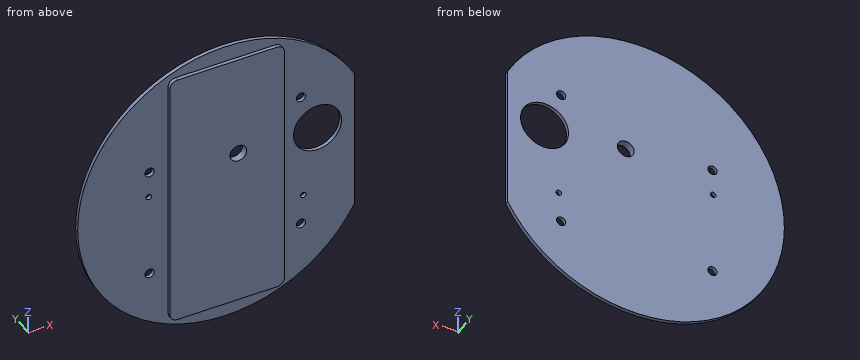
from build123d import *

# Parameters (mm, degrees)
F1_DEPTH  = 2
F2_W      = 62
F2_H      = 142.5
F3_DEPTH  = 2
F4_R      = 4
F5_R      = 4.5
F6_DEPTH  = 4
F7_R      = 13
F8_DEPTH  = 2
F9_R      = 2.5
F10_DEPTH = 2
F11_R     = 1.5
F12_DEPTH = 2


with BuildPart() as f1:
    # F0 (on Front) → F1 (new body)
    with BuildSketch(Plane.XZ):
        with BuildLine():
            ThreePointArc((70, 38.729833), (-80, 0), (70, -38.729833))
            Line((70, -38.729833), (70, 38.729833))
        make_face()
    extrude(amount=F1_DEPTH)

    # F2 (on face) → F3 (join)
    with BuildSketch(Plane.XZ.offset(2)):
        Rectangle(F2_W, F2_H)
    extrude(amount=F3_DEPTH)

    # F4
    f4_edges = [f1.edges().sort_by_distance(p)[0] for p in [
        (-31, -3, -71.25),
        (31, -3, -71.25),
        (31, -3, 71.25),
        (-31, -3, 71.25),
    ]]
    fillet(f4_edges, radius=F4_R)

    # F5 (on face) → F6 (cut)
    with BuildSketch(Plane.XZ.offset(4)):
        with Locations((6, 15.75)):
            Circle(F5_R)
    extrude(amount=-F6_DEPTH, mode=Mode.SUBTRACT)

    # F7 (on face) → F8 (cut)
    with BuildSketch(Plane.XZ.offset(2)):
        with Locations((50, 13.729833)):
            Circle(F7_R)
    extrude(amount=-F8_DEPTH, mode=Mode.SUBTRACT)

    # F9 (on face) → F10 (cut)
    with BuildSketch(Plane.XZ.offset(2)):
        with Locations((-41, 20)):
            Circle(F9_R)
        with Locations((-41, -40)):
            Circle(F9_R)
        with Locations((41, 35)):
            Circle(F9_R)
        with Locations((41, -40)):
            Circle(F9_R)
    extrude(amount=-F10_DEPTH, mode=Mode.SUBTRACT)

    # F11 (on face) → F12 (cut)
    with BuildSketch(Plane.XZ.offset(2)):
        with Locations((-41.405737, 5.505678)):
            Circle(F11_R)
        with Locations((42.2996, -23.55126)):
            Circle(F11_R)
    extrude(amount=-F12_DEPTH, mode=Mode.SUBTRACT)


solid = f1.part
Can you work these out from the model? Positions are in its coordinate system, mm. Coordinates: 2 decimals unless noted, no trailing zeros. Order: outer loops, then holes, each group sorted by start corner. A loop starts at its lowest first (then second) coordinate and runs counter-clockwise, first axis right, second up. Notation, with made-up numbers: (-8, -23) -> (8, -23) arc R23 ccw to (8, 11) -> close; hole circle Ø2 at (8.25, -30). An arc over 180 degrees is marked (long way). Use one line per item in the form item = value.
Q1. Imagine slicing it at D-D, the plane z = -15. List the corners of the cut face in (x, y) for me, then the cut area to 3 significant figures.
From the geometry:
outline = (-78.58, -2) -> (-31, -2) -> (-31, -4) -> (31, -4) -> (31, -2) -> (70, -2) -> (70, 0) -> (-78.58, 0) -> close
area = 421 mm²
Q2. Imagine slicing it at A-A, the plane x = 6. List the corners of the cut face in (y, z) for me.
From the geometry:
outline = (-4, -71.25) -> (-2, -71.25) -> (-2, -79.77) -> (0, -79.77) -> (0, 11.25) -> (-4, 11.25) -> close; (-4, 20.25) -> (0, 20.25) -> (0, 79.77) -> (-2, 79.77) -> (-2, 71.25) -> (-4, 71.25) -> close
Q3. Imagine slicing it at B-B, the plane z = 35. List the corners of the cut face in (x, y) for me.
From the geometry:
outline = (-71.94, -2) -> (-31, -2) -> (-31, -4) -> (31, -4) -> (31, -2) -> (38.5, -2) -> (38.5, 0) -> (-71.94, 0) -> close; (43.5, -2) -> (70, -2) -> (70, 0) -> (43.5, 0) -> close
Q4. Will these pins go through, and if not, where does the flat tip stop? P1, Ø4.5, axis at x = -41, z = 20, coming from the -Y side; P2, Ø1.5, axis at y = -3.5, z = -23, coming from the -X side; P3, Ø3.5, axis at x = 42.3, z = -23.55, coming from the -Y side; P4, Ø2, axis at x = -35, y = -1, coming from the +Z side.
From the geometry:
P1 = through
P2 = -31
P3 = -2
P4 = 72.42
Q5. I need wall thicknesses on L1, parallel to X at y = -1.6, z = 14; L2, parallel to X at y = -2.85, z = -5; L3, parallel to Z at x = 51.5, y = -0.35. Which ranges of each line are inside material? Lowest first, please.
From the geometry:
L1 = -78.77 to 1.85, 10.15 to 37, 63 to 70
L2 = -31 to 31
L3 = -61.22 to 0.82, 26.64 to 61.22
Q6. Imagine slicing it at C-C, the plane y = -3.4. List the corners of the cut face in (x, z) for me, then the cut area to 3 significant figures.
From the geometry:
outline = (-31, -67.25) arc R4 ccw to (-27, -71.25) -> (27, -71.25) arc R4 ccw to (31, -67.25) -> (31, 67.25) arc R4 ccw to (27, 71.25) -> (-27, 71.25) arc R4 ccw to (-31, 67.25) -> close; hole circle Ø9 at (6, 15.75)
area = 8,760 mm²
